from build123d import *

# Parameters (mm, degrees)
SKETCH1_R                          = 52.5
SKETCH1_R_2                        = 50.5
MAIN_BLADE_CASE_EXTRUDE_DEPTH      = 41
SKETCH2_R                          = 50.5
EXTRUDE_FOR_GOBLET_TO_SIT_ON_DEPTH = 9
SKETCH5_R                          = 15
SKETCH4_R                          = 25
SKETCH8_R                          = 33
SKETCH8_R_2                        = 32
MAIN_LOWER_EXTRUDE_DEPTH           = 10
SKETCH9_R                          = 32
SKETCH9_R_2                        = 25
SECOND_LOWER_EXTRUDE_DEPTH         = 6
SKETCH12_R                         = 25
THIRD_LOWER_EXTRUDE_DEPTH          = 5
SKETCH13_R                         = 1
HOLE_FOR_SCREW_BLADE_CASING_DEPTH  = 89


with BuildPart() as part:
    # Sketch1 → Main Blade Case Extrude (new body)
    with BuildSketch(Plane(origin=(0, 0, 0), x_dir=(1, 0, 0), z_dir=(0, 1, 0))):
        with Locations(Location((0, 0, 0), (0, 0, 270))):
            Circle(SKETCH1_R)
        with Locations(Location((0, 0, 0), (0, 0, 270))):
            Circle(SKETCH1_R_2, mode=Mode.SUBTRACT)
    extrude(amount=MAIN_BLADE_CASE_EXTRUDE_DEPTH)

    # Sketch2 → Extrude for Goblet to Sit On (add)
    with BuildSketch(Plane(origin=(0, 21, 0), x_dir=(-1, 0, 0), z_dir=(0, -1, 0))):
        with Locations(Location((0, 0, 0), (0, 0, 90))):
            Circle(SKETCH2_R)
    extrude(amount=-EXTRUDE_FOR_GOBLET_TO_SIT_ON_DEPTH)

    # Sketch5 → Rounded Middle Section section 0
    with BuildSketch(Plane(origin=(0, 35, 0), x_dir=(1, 0, 0), z_dir=(0, 1, 0))):
        Circle(SKETCH5_R)
    # Sketch4 → Rounded Middle Section section 1
    with BuildSketch(Plane(origin=(0, 30, 0), x_dir=(1, 0, 0), z_dir=(0, 1, 0))):
        Circle(SKETCH4_R)
    loft()

    # Sketch8 → Main Lower Extrude (add)
    with BuildSketch(Plane.XZ.offset(-21)):
        with Locations(Location((0, 0, 0), (0, 0, 270))):
            Circle(SKETCH8_R)
        with Locations(Location((0, 0, 0), (0, 0, 270))):
            Circle(SKETCH8_R_2, mode=Mode.SUBTRACT)
    extrude(amount=MAIN_LOWER_EXTRUDE_DEPTH)

    # Sketch9 → Second Lower Extrude (add)
    with BuildSketch(Plane.XZ.offset(-21)):
        with Locations(Location((0, 0, 0), (0, 0, 270))):
            Circle(SKETCH9_R)
        with Locations(Location((0, 0, 0), (0, 0, 270))):
            Circle(SKETCH9_R_2, mode=Mode.SUBTRACT)
    extrude(amount=SECOND_LOWER_EXTRUDE_DEPTH)

    # Sketch12 → Third Lower Extrude (add)
    with BuildSketch(Plane(origin=(0, 21, 0), x_dir=(-1, 0, 0), z_dir=(0, -1, 0))):
        with Locations(Location((0, 0, 0), (0, 0, 90))):
            Circle(SKETCH12_R)
    extrude(amount=THIRD_LOWER_EXTRUDE_DEPTH)

    # Sketch13 → Hole for Screw (Blade Casing) (cut)
    with BuildSketch(Plane.XZ.offset(-16)):
        with Locations(Location((0, 0, 0), (0, 0, 270))):
            Circle(SKETCH13_R)
    extrude(amount=-HOLE_FOR_SCREW_BLADE_CASING_DEPTH, mode=Mode.SUBTRACT)


solid = part.part
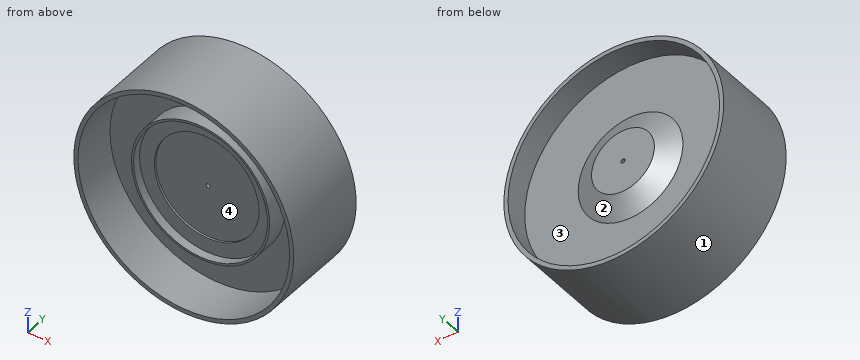
Source: CAD feature listing. Evaluate the final solid. Frame: model axes, mm. Face numbers are marked on the shaded views. A direction names the side the tool comes from. Give positions to 0.01 mm unless a question says otherwise; leave off trailing zeros. Write each loop counter-clockwise with the first axis right and the second up, starting at its lowest first coordinate (ties: lowest second). Pieces come first, ordered by that corner, then holes. Notation, with made-up numbers: M -39.75,22.25 L -8.75,22.25 A13 cw -8.75,31.25 Z; hole C 88,47 d3. An arc over 180 degrees is marked long. Return JSON: item names as keys, results as strings. Group by question number.
1) Cut plane A-A, the plane y = 17.5. Output: boundary loops of the cut face in (x, z).
2) Draft query along X for the marked faces 1 and 2. Return one class per face: released by +X, released by -X, zero draft, split by the parting line, or undercut.
3) First-contact query: pin 1 Ø5 at (y, z) = (30, 10.5) entering from -X; pin 2 Ø20 at (x, z) = (-11.5, -3.5) entering from -Y; pin 3 Ø5 at (x, z) = (4.5, 23) entering from +Y; pin 4 Ø10 at (x, z) = (-32, -38) entering from +Y. Flat tips, straight axial feed; report the tip coordinate or a pass-through.
4) Cut plane D-D, the plane x = -39.5. Output: boundary loops of the cut face in (y, z).
5) Set-up query: the marked faces 3 and 4. Return all of +Z, -Z, +X, -X, +Y, -Y with unobstructed straight access to the full face (end or side cutting, diameter ignored); none if empty.
6) Ray query, L1, parallel to X at y = 37, z = 0; L2, parallel to Z at x = -10, y = 18.5; L3, parallel to Z at x = -11, y = 33. Return the intervals inside material, ascending.
7) Cut plane B-B, the plane y = 38. Output: boundary loops of the cut face in (x, z), then the cut area to 3 significant figures.
8) Cut plane C-C, the plane z = -39. Output: boundary loops of the cut face in (x, y).
Data:
{
 "1": {"outline": "C 0,0 d105; C 0,0 d66; hole C 0,0 d101; hole C 0,0 d2"},
 "2": {"face 1": "split by the parting line", "face 2": "undercut"},
 "3": {"pin 1": "stops at x = -51.89", "pin 2": "stops at y = 16", "pin 3": "stops at y = 32.03", "pin 4": "stops at y = 41"},
 "4": {"outline": "M 0,-34.58 L 41,-34.58 L 41,-31.46 L 30,-31.46 L 30,31.46 L 41,31.46 L 41,34.58 L 0,34.58 L 0,31.46 L 21,31.46 L 21,-31.46 L 0,-31.46 Z"},
 "5": {"face 3": "+Y", "face 4": "-Y"},
 "6": {"L1": "x = -52.5 to -50.5, 50.5 to 52.5", "L2": "z = -51.54 to -49.5, -31.45 to 31.45, 49.5 to 51.54", "L3": "z = -51.33 to -49.29, -15.49 to 15.49, 49.29 to 51.33"},
 "7": {"outline": "C 0,0 d105; hole C 0,0 d101", "area": "647 mm²"},
 "8": {"outline": "M -35.15,0 L -32.08,0 L -32.08,21 L 32.08,21 L 32.08,0 L 35.15,0 L 35.15,41 L 32.08,41 L 32.08,30 L -32.08,30 L -32.08,41 L -35.15,41 Z"}
}
